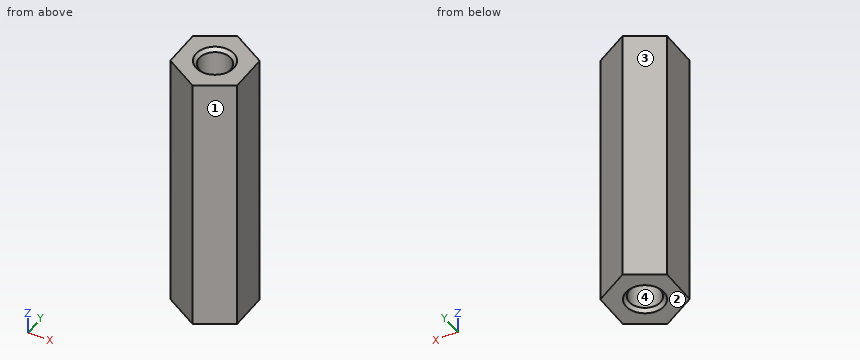
from build123d import *

# Parameters (mm, degrees)
SKETCH1_R           = 2.35
BOSS_EXTRUDE1_DEPTH = 40
CHAMFER4_SIZE       = 0.5


with BuildPart() as part:
    # Sketch1 → Boss-Extrude1 (new body)
    with BuildSketch(Plane(origin=(0, 0, 0), x_dir=(-1, 0, 0), z_dir=(0, 0, -1))):
        Polygon((-5.000000075, 2.886751389), (-5.000000075, -2.886751389), (0, -5.773502778), (5.000000075, -2.886751389), (5.000000075, 2.886751389), (0, 5.773502778), align=None)
        Circle(SKETCH1_R, mode=Mode.SUBTRACT)
    extrude(amount=-BOSS_EXTRUDE1_DEPTH)

    # Chamfer4
    chamfer4_edges = [part.edges().sort_by_distance(p)[0] for p in [
        (2.35, 0, 40),
        (2.35, 0, 0),
    ]]
    chamfer(chamfer4_edges, length=CHAMFER4_SIZE)


solid = part.part
Here's how the part is built. I have some questions about the finished solid (model axes, mm). Face numbers are marked on the shaded views. Give positions to 0.01 mm unless a question says otherwise; leave off trailing zeros. Write each loop counter-clockwise with the first axis right and the second up, starting at its lowest first coordinate (ties: lowest second). Pieces come first, ordered by that corner, then holes. Notation, with made-up numbers: (10.5, 14) -> (15.5, 14) arc R37 cw to (15.5, 50) -> close; hole circle Ø4 at (65, 1). An arc over 180 degrees is marked (long way). Use one line per item in the form item = value. Start each with the question number.
1. Imagine slicing it at C-C on y = -3.5. List the corners of the cut face in (x, z) for me, plus the area to 3 significant figures.
2. Thinking about a two-plate mould opening in Y: for the marked faces 1, 2, 3 and 4, which applies, +Y half, -Y half, draft (parallel to the pull), parting line (faces both ways), or undercut?
3. Will these pins go through, and if not, where does the flat tip stop? pin 1 Ø5.5 at (x, y) = (0, 0) entering from -Z; pin 2 Ø2 at (y, z) = (-4, 9.5) entering from +X.
4. Imagine slicing it at A-A on y = 0. List the corners of the cut face in (x, z) for me, plus the area to 4 significant figures.
5. If I drill on L1, parallel to Y at x = 0, z = 26; L2, parallel to Y at x = -1, z = 17; L3, parallel to X at y = -0.25, z = 8.5, over which ranges is the centre line in solid material (lowest first)?
6. Imagine slicing it at D-D on x = 3.25. List the corners of the cut face in (y, z) for me, plus the area to 3 significant figures.
7. Imagine slicing it at B-B on z = 5. List the corners of the cut face in (x, y) for me, plus the area to 3 significant figures.
Entries:
q1.outline = (-3.94, 0) -> (3.94, 0) -> (3.94, 40) -> (-3.94, 40) -> close
q1.area = 315 mm²
q2.face_1 = -Y half
q2.face_2 = draft
q2.face_3 = +Y half
q2.face_4 = undercut
q3.pin_1 = 0.1
q3.pin_2 = 4.8
q4.outline = (-5, 0) -> (-2.85, 0) -> (-2.35, 0.5) -> (-2.35, 39.5) -> (-2.85, 40) -> (-5, 40) -> close; (2.35, 0.5) -> (2.85, 0) -> (5, 0) -> (5, 40) -> (2.85, 40) -> (2.35, 39.5) -> close
q4.area = 211.5 mm²
q5.L1 = -5.77 to -2.35, 2.35 to 5.77
q5.L2 = -5.2 to -2.13, 2.13 to 5.2
q5.L3 = -5 to -2.34, 2.34 to 5
q6.outline = (-3.9, 0) -> (3.9, 0) -> (3.9, 40) -> (-3.9, 40) -> close
q6.area = 312 mm²
q7.outline = (-5, -2.89) -> (0, -5.77) -> (5, -2.89) -> (5, 2.89) -> (0, 5.77) -> (-5, 2.89) -> close; hole circle Ø4.7 at (0, 0)
q7.area = 69.3 mm²
